Build history of the part. All positions in model axes, mm. A direction names the side the tool comes from. Round coordinates to 2 decimals unless told otherwise and drop trailing zeros. Loops run counter-clockwise (first coordinate to the right, second up) from the corner with the lowest first, then second, coordinate; pieces in that order, holes last.
from build123d import *

# Parameters (mm, degrees)
F0_W      = 60
F0_H      = 5
F1_DEPTH  = 3
F2_W      = 15
F2_H      = 5
F3_DEPTH  = 6
F4_R      = 5.25
F5_DEPTH  = 5
F6_DEPTH  = 3
F8_DEPTH  = 3
F9_R      = 1.5
F10_DEPTH = 25
F11_R     = 2


with BuildPart() as f1:
    # F0 (on Top) → F1 (new body)
    with BuildSketch(Plane.XY):
        Rectangle(F0_W, F0_H)
    extrude(amount=F1_DEPTH)

    # F2 (on face) → F3 (join)
    with BuildSketch(Plane.XY.offset(3)):
        with Locations((-22.5, 5)):
            Rectangle(F2_W, F2_H)
        with Locations((-22.5, 0)):
            Rectangle(F2_W, F2_H)
        with Locations((-22.5, -5)):
            Rectangle(F2_W, F2_H)
    extrude(amount=-F3_DEPTH)

    # F4 (on face) → F5 (cut)
    with BuildSketch(Plane(origin=(0, 0, -3), x_dir=(1, 0, 0), z_dir=(0, 0, -1))):
        with Locations((-22.5, 0)):
            Circle(F4_R)
    extrude(amount=-F5_DEPTH, mode=Mode.SUBTRACT)

    # F6 (cut): a face of the model
    f6_faces = [f1.faces().sort_by_distance(p)[0] for p in [
        (-30, 0, 0),
    ]]
    extrude(f6_faces, amount=-F6_DEPTH, mode=Mode.SUBTRACT)

    # F7 (on face) → F8 (join)
    with BuildSketch(Plane(origin=(0, 0, 0), x_dir=(1, 0, 0), z_dir=(0, 0, -1))):
        with BuildLine():
            ThreePointArc((23.4616515847, -2.5), (31.2711335675, -6.8836196477), (37, 0))
            ThreePointArc((37, 0), (31.2711335675, 6.8836196477), (23.4616515847, 2.5))
            Line((23.4616515847, 2.5), (30, 2.5))
            Line((30, 2.5), (30, -2.5))
            Line((30, -2.5), (23.4616515847, -2.5))
        make_face()
        with BuildLine():
            Line((30, 2.5), (23.4616515847, 2.5))
            ThreePointArc((23.4616515847, 2.5), (23, 0), (23.4616515847, -2.5))
            Line((23.4616515847, -2.5), (30, -2.5))
            Line((30, -2.5), (30, 2.5))
        make_face()
    extrude(amount=-F8_DEPTH)

    # F9 (on face) → F10 (cut)
    with BuildSketch(Plane(origin=(0, 0, 0), x_dir=(1, 0, 0), z_dir=(0, 0, -1))):
        with Locations((30, 0)):
            Circle(F9_R)
    extrude(amount=-F10_DEPTH, mode=Mode.SUBTRACT)

    # F11
    f11_edges = [f1.edges().sort_by_distance(p)[0] for p in [
        (-15, -7.5, 0),
        (-15, 7.5, 0),
    ]]
    fillet(f11_edges, radius=F11_R)


solid = f1.part
(1) Pull direction Y, two halves, no side cores. Call faces 6 (the face through (-27, 0.1, 2.7)), 7 (the face through (-22, 0, 2)), 8 (the face through (4, 2.5, 1)): +Y half, -Y half, draft (parallel to the pull), parting line (faces both ways), or undercut.
Responses:
face 6: draft
face 7: undercut
face 8: +Y half
(2) Slice it at C-C on x = -22.5. List the corners of the cut face in (y, z), plus the area to 3 significant figures.
Responses:
outline: (-7.5, -3) - (-5.25, -3) - (-5.25, 2) - (5.25, 2) - (5.25, -3) - (7.5, -3) - (7.5, 3) - (-7.5, 3) - close
area: 37.5 mm2
(3) Which spindle directions (+Z, -Z, +X, -X, +Y, -Y) get a long thin tool onto all of the face, cutting with end or side? Do faces 1 (the face through (-17.253, 0.191, -0.535)), 2 (the face through (-17, 0, -3)), 3 (the face through (-15.57, 6.9, -0.04)), 4 (the face through (4, -2.5, 1)), 5 (the face through (16, 0, 0)). Say none if no direction does.
Responses:
face 1: -Z
face 2: -Z, +X, -X, +Y, -Y
face 3: +Z, -Z, +Y
face 4: +Z, -Z, -Y
face 5: -Z, +X, +Y, -Y
(4) Slice it at D-D on z = 0.8. List the corners of the cut face in (x, y), plus the area to 3 significant figures.
Responses:
outline: (-27, -7.5) - (-17, -7.5) arc R2 ccw to (-15, -5.5) - (-15, -2.5) - (23.46, -2.5) arc R7 ccw (long way) to (23.46, 2.5) - (-15, 2.5) - (-15, 5.5) arc R2 ccw to (-17, 7.5) - (-27, 7.5) - (-27, 2.7) arc R5.25 cw (long way) to (-27, -2.7) - close; hole circle Ø3 at (30, 0)
area: 432 mm2
(5) Probe line 1 (Y direction, x = 30, z = 2.4); line 2 (Y direction, x = -22.5, z = -1.65); line 3 (Z direction, x = 0.5, y = 1.25). List the from-to ranges inside material, lowest first.
Responses:
line 1: y = -7 to -1.5, 1.5 to 7
line 2: y = -7.5 to -5.25, 5.25 to 7.5
line 3: z = 0 to 3
(6) Pin check, flat tips, straight feed: P1, Ø1.5, axis at x = 13, z = 1.5, coming from the +Y side; P2, Ø5, axis at x = -24.5, y = -0.5, coming from the -Z side; P3, Ø1.5, axis at x = 13, z = 2, coming from the -Y side. Stop position of each tip, or through.
Responses:
P1: stops at y = 2.5
P2: stops at z = 2
P3: stops at y = -2.5
(7) Slice it at A-A on x = 30. List the corners of the cut face in (y, z), plus the area to 3 significant figures.
Responses:
outline: (-7, 0) - (-1.5, 0) - (-1.5, 3) - (-7, 3) - close; (1.5, 0) - (7, 0) - (7, 3) - (1.5, 3) - close
area: 33.0 mm2
(8) Slice it at B-B on y = 4.5. List the corners of the cut face in (x, z).
Responses:
outline: (-27, -3) - (-25.2, -3) - (-25.2, 2) - (-19.8, 2) - (-19.8, -3) - (-15, -3) - (-15, 3) - (-27, 3) - close; (24.64, 0) - (35.36, 0) - (35.36, 3) - (24.64, 3) - close
